from build123d import *

# Parameters (mm, degrees)
F1_DEPTH = 0.5


with BuildPart() as f1:
    # F0 (on Top) → F1 (new body)
    with BuildSketch(Plane.XY):
        Polygon((0, 10), (-10, 10), (-10, 0), (-1.480661, 0), (0, 0), (0, 1.480661), align=None)
        with BuildLine():
            ThreePointArc((-1.480661, 0), (1.046985, -1.046985), (0, 1.480661))
            Line((0, 1.480661), (0, 0))
            Line((0, 0), (-1.480661, 0))
        make_face()
    extrude(amount=F1_DEPTH)


solid = f1.part
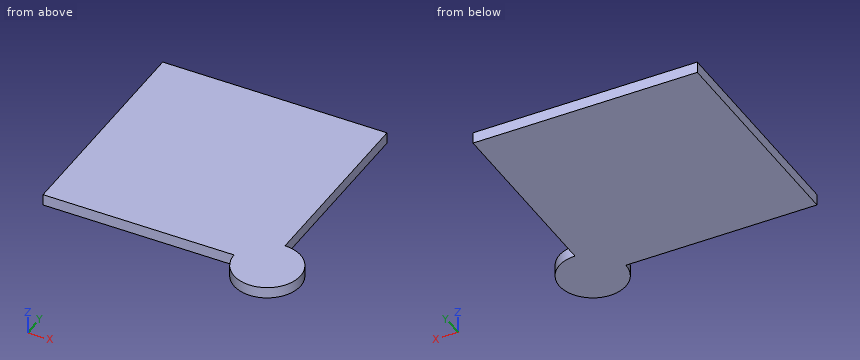
Model file for the job. Use its own axes, mm. Give positions to 0.01 mm unless a question says otherwise; leave off trailing zeros. Loops run counter-clockwise (first coordinate to the right, second up) from the corner with the lowest first, then second, coordinate; pieces in that order, holes last.
Item 1: Drill centre lines: line 1 along Y through (x, z) = (-8, 0.4); line 2 along X through (y, z) = (3.25, 0.45); line 3 along Y through (x, z) = (1, 0.25). Where is each one in solid material? Low to high.
Check values:
line 1: y = 0 to 10
line 2: x = -10 to 0
line 3: y = -1.09 to 1.09
Item 2: Slice it at C-C (y = 5). Write the cut outline in (x, z).
Check values:
outline: (-10, 0) - (0, 0) - (0, 0.5) - (-10, 0.5) - close
Item 3: Slice it at A-A (z = 0.3). Write the cut outline in (x, y).
Check values:
outline: (-10, 0) - (-1.48, 0) arc R1.48 ccw (long way) to (0, 1.48) - (0, 10) - (-10, 10) - close
Item 4: Slice it at B-B (x = -3). Write the cut outline in (y, z).
Check values:
outline: (0, 0) - (10, 0) - (10, 0.5) - (0, 0.5) - close
